Here's the drawing with two shaded views (mm, measured from the low corner). I have some questions. A direction names the side the tool comes from. Coordinates: 2 decimals unless noted, no trailing zeros. Write each loop counter-clockwise with the first axis right and the second up, starting at its lowest first coordinate (ties: lowest second). Pieces come first, ordered by that corner, then holes.
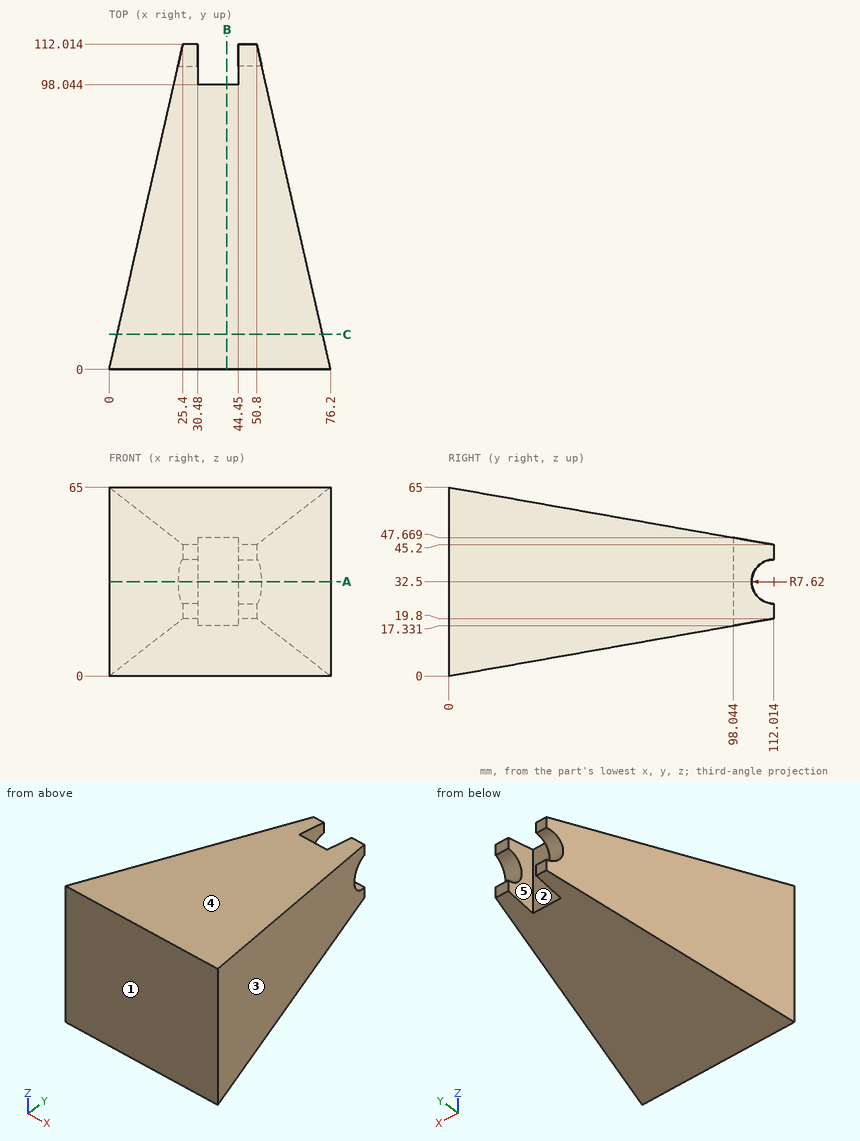
1. I want a section at B-B on x = 40.5. Please give me the cut outline in (y, z), plus the area to 3 significant figures.
Verdict:
outline: (0, 0) - (98.04, 17.33) - (98.04, 47.67) - (0, 65) - close
area: 4,670 mm2
2. I want a section at C-C on y = 12. Please give me the cut outline in (x, z).
Verdict:
outline: (2.72, 2.12) - (73.48, 2.12) - (73.48, 62.88) - (2.72, 62.88) - close
3. On a 3-axis mill with a long thin cutter (end or side, diameter ignored), from which of +Z, -Z, +X, -X, +Y, -Y can I reach the whole of each face in a straight line? I mean the marked faces 4 and 5. Say none if no direction works.
Verdict:
face 4: +Z, +X, -X, +Y
face 5: +Z, -Z, +Y
4. If we mould it in two halves opening along X, with no side actions, what happens to the marked faces 1, 2 and 3? For each: pulls with the +X half, pulls with the -X half, needs draft (parallel to the pull), parting line crosses it, or undercut.
Verdict:
face 1: needs draft
face 2: undercut
face 3: pulls with the +X half
5. I want a section at A-A on z = 32.5. Please give me the cut outline in (x, y).
Verdict:
outline: (0, 0) - (76.2, 0) - (52.53, 104.39) - (44.45, 104.39) - (44.45, 98.04) - (30.48, 98.04) - (30.48, 104.39) - (23.67, 104.39) - close
6. Please list where these lines run through material, in increasing order: line 1 along X through (y, z) = (93, 44.5); line 2 along Y through (x, z) = (46.5, 27.5) (1 decimal); line 3 along X through (y, z) = (25, 60.5).
Verdict:
line 1: x = 21.09 to 55.11
line 2: y = 0 to 106.3
line 3: x = 5.67 to 70.53
7. For pin 1 (1.5 mm diameter, centred on x = 45.5, y = 51, fed in from -Z); pin 2 (4 mm diameter, centred on x = 68, y = 48.5, fed in from -Z); pin 3 (7 mm diameter, centred on y = 102, z = 33.5, fed in from +X) (1 decimal); pin 4 (3 mm diameter, centred on x = 56, y = 20.5, fed in from +Z), each with a flat end and sliding along its axis, tell me the tip position at first contact or that it passes through.
Verdict:
pin 1: stops at z = 8.88
pin 2: passes through
pin 3: stops at x = 53.9
pin 4: stops at z = 61.64
